from build123d import *

# Parameters (mm, degrees)
SKETCH7_R            = 15
BOSS_EXTRUDE2_DEPTH  = 12
SKETCH9_R            = 11
CUT_EXTRUDE1_DEPTH   = 4
SKETCH8_R            = 7.5
CUT_EXTRUDE2_DEPTH   = 20
BOSS_EXTRUDE4_START  = -3
SKETCH11_W           = 5
SKETCH11_H           = 10
BOSS_EXTRUDE4_DEPTH  = 48
SKETCH14_W           = 5
SKETCH14_H           = 10
BOSS_EXTRUDE5_DEPTH  = 6.3
SKETCH17_W           = 2.5
SKETCH17_H           = 10
BOSS_EXTRUDE8_DEPTH  = 15
SKETCH20_R           = 1.5
CUT_EXTRUDE3_DEPTH   = 15
FILLET2_R            = 2
FILLET7_R            = 0.5
FILLET8_R            = 0.5
FILLET2_OF_MIRROR5_R = 2


with BuildPart() as part:
    # Sketch7 → Boss-Extrude2 (new body)
    with BuildSketch(Plane.XY.offset(37)):
        Circle(SKETCH7_R)
    extrude(amount=-BOSS_EXTRUDE2_DEPTH)

    # Sketch9 → Cut-Extrude1 (cut)
    with BuildSketch(Plane.XY.offset(33)):
        Circle(SKETCH9_R)
    extrude(amount=-CUT_EXTRUDE1_DEPTH, mode=Mode.SUBTRACT)

    # Sketch8 → Cut-Extrude2 (cut)
    with BuildSketch(Plane.XY.offset(37)):
        Circle(SKETCH8_R)
    extrude(amount=-CUT_EXTRUDE2_DEPTH, mode=Mode.SUBTRACT)

    # Sketch11 → Boss-Extrude4 (add)
    with BuildSketch(Plane(origin=(15, 0, 0), x_dir=(0, 0, -1), z_dir=(1, 0, 0)).offset(BOSS_EXTRUDE4_START)):
        with Locations((-31.203319291, 0.070417763)):
            Rectangle(SKETCH11_W, SKETCH11_H)
    boss_extrude4 = extrude(amount=BOSS_EXTRUDE4_DEPTH)

    # Sketch14 → Boss-Extrude5 (add)
    with BuildSketch(Plane.XY.offset(33.703319291)):
        with Locations((57.5, 0.070417763)):
            Rectangle(SKETCH14_W, SKETCH14_H)
    boss_extrude5 = extrude(amount=BOSS_EXTRUDE5_DEPTH)

    # Sketch17 → Boss-Extrude8 (add)
    with BuildSketch(Plane.XY.offset(40.003319291)):
        with Locations((56.25, 0.070417763)):
            Rectangle(SKETCH17_W, SKETCH17_H)
    boss_extrude8 = extrude(amount=BOSS_EXTRUDE8_DEPTH)

    # Sketch20 → Cut-Extrude3 (cut)
    with BuildSketch(Plane(origin=(57.5, 0, 0), x_dir=(0, 0, -1), z_dir=(1, 0, 0))):
        with Locations((-44.003319291, 0)):
            Circle(SKETCH20_R)
        with Locations((-51.003319291, 0)):
            Circle(SKETCH20_R)
    cut_extrude3 = extrude(amount=-CUT_EXTRUDE3_DEPTH, mode=Mode.SUBTRACT)

    # Fillet2
    fillet2_edges = [part.edges().sort_by_distance(p)[0] for p in [
        (14.166835178, -4.929582237, 31.203319291),
        (14.777611852, 2.573361217, 28.703319291),
        (14.117041606, 5.070417763, 31.203319291),
        (14.777611852, 2.573361217, 33.703319291),
    ]]
    fillet(fillet2_edges, radius=FILLET2_R)

    # Fillet7
    fillet7_edges = [part.edges().sort_by_distance(p)[0] for p in [
        (-15, 0, 37),
    ]]
    fillet(fillet7_edges, radius=FILLET7_R)

    # Fillet8
    fillet8_edges = [part.edges().sort_by_distance(p)[0] for p in [
        (-15, 0, 25),
    ]]
    fillet(fillet8_edges, radius=FILLET8_R)

    # Mirror5: Boss-Extrude4, Boss-Extrude5, Boss-Extrude8, Cut-Extrude3 across plane
    add(boss_extrude4.mirror(Plane(origin=(0, 0, 0), x_dir=(0, 0, 1), z_dir=(1, 0, 0))))
    add(boss_extrude5.mirror(Plane(origin=(0, 0, 0), x_dir=(0, 0, 1), z_dir=(1, 0, 0))))
    add(boss_extrude8.mirror(Plane(origin=(0, 0, 0), x_dir=(0, 0, 1), z_dir=(1, 0, 0))))
    add(cut_extrude3.mirror(Plane(origin=(0, 0, 0), x_dir=(0, 0, 1), z_dir=(1, 0, 0))), mode=Mode.SUBTRACT)

    # Fillet2 of Mirror5
    fillet2_of_mirror5_edges = [part.edges().sort_by_distance(p)[0] for p in [
        (-14.166835178, -4.929582237, 31.203319291),
        (-14.777611852, 2.573361217, 28.703319291),
        (-14.117041606, 5.070417763, 31.203319291),
        (-14.777611852, 2.573361217, 33.703319291),
    ]]
    fillet(fillet2_of_mirror5_edges, radius=FILLET2_OF_MIRROR5_R)


solid = part.part
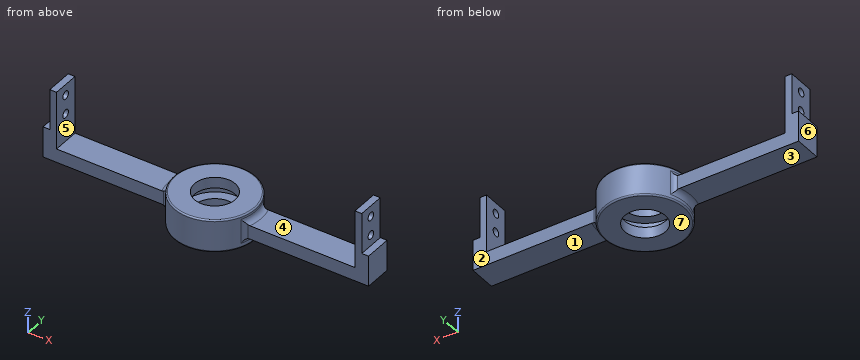
CAD build for the part. Positions are in the model's coordinates, mm. Face numbers are marked on the shaded views. A direction names the side the tool comes from. Coordinates: 2 decimals unless noted, no trailing zeros. Loops run counter-clockwise (first coordinate to the right, second up) from the corner with the lowest first, then second, coordinate; pieces in that order, holes last. Notation, with made-up numbers: (88, 82) - (123, 82) arc R17 cw to (123, 97) - close; hole circle Ø4 at (-16.5, 12). An arc over 180 degrees is marked (long way). Use one line per item in the form item = value. Start each with the question number.
1) Flat gauge pins, fed straight in: pin 1 (5 mm diameter, centred on y = -6, z = 44.5, fed in from +X); pin 2 (8 mm diameter, centred on x = -46.5, y = 4.5, fed in from -Z); pin 3 (5 mm diameter, centred on y = 8, z = 43, fed in from -X); pin 4 (11 mm diameter, centred on y = 2, z = 48.5, fed in from -X). Where does each tip first touch, or does it go through?
2) Band-saw the part on D-D (x = 41). Give the cut face in (y, z), and give its area (3 significant figures).
3) Band-saw the part on C-C (y = 0). State how many separate pieces and enclosed holes the cut face has, and give its area (3 significant figures).
4) Two-plate mould, pull along X, no slides. Class the marked faces 5, 6 and 7: +X half, -X half, draft (parallel to the pull), parting line (faces both ways), or undercut.
5) Band-saw the part on A-A (x = 0). Give the cut face in (y, z).
6) Tool access for the marked faces 1, 2, 3 and 4: list every direction of +Z, -Z, +X, -X, +Y, -Y with a clear straight run to the whole face (end or side of a thin tool).
7) Band-saw the part on B-B (z = 48). Give the cut face in (x, y).
8) Drill centre lines: L1, parallel to Z at x = -56.35, y = 0; L2, parallel to Y at x = 0, z = 26.35; L3, parallel to Z at x = 9, y = -4. Where is each one in solid material? Low to high. Write a range as from..to.
Check values:
q1.pin_1 = 57.5
q1.pin_2 = 28.7
q1.pin_3 = through
q1.pin_4 = -57.5
q2.outline = (-4.93, 28.7) - (5.07, 28.7) - (5.07, 33.7) - (-4.93, 33.7) - close
q2.area = 50.0 mm2
q3.separate_pieces = 6
q3.enclosed_holes = 0
q3.area = 713 mm2
q4.face_5 = undercut
q4.face_6 = -X half
q4.face_7 = draft
q5.outline = (-15, 25.5) arc R0.5 ccw to (-14.5, 25) - (-7.5, 25) - (-7.5, 29) - (-11, 29) - (-11, 33) - (-7.5, 33) - (-7.5, 37) - (-14.5, 37) arc R0.5 ccw to (-15, 36.5) - close; (7.5, 25) - (14.5, 25) arc R0.5 ccw to (15, 25.5) - (15, 36.5) arc R0.5 ccw to (14.5, 37) - (7.5, 37) - (7.5, 33) - (11, 33) - (11, 29) - (7.5, 29) - close
q6.face_1 = -Z, +X, +Y, -Y
q6.face_2 = +Z, -Z, +X, +Y
q6.face_3 = -Z, -X, +Y, -Y
q6.face_4 = +Z, +Y, -Y
q7.outline = (-57.5, -4.93) - (-55, -4.93) - (-55, 5.07) - (-57.5, 5.07) - close; (55, -4.93) - (57.5, -4.93) - (57.5, 5.07) - (55, 5.07) - close
q8.L1 = 28.7..42.5, 45.5..49.5, 52.5..55
q8.L2 = -15..-7.5, 7.5..15
q8.L3 = 25..29, 33..37
